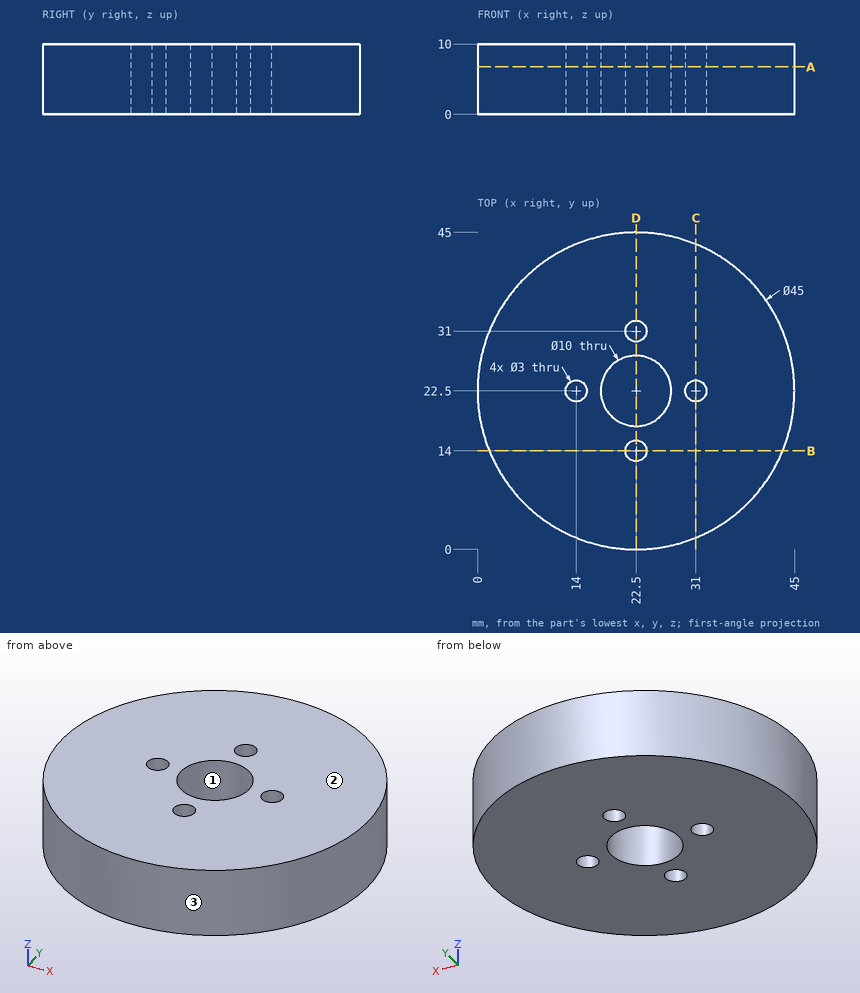
Geometry check sheet. Reference: drawing and pictorial views, mm from the part's lowest x, y, z. Give positions to 0.01 mm unless a question says otherwise; leave off trailing zeros. Order: outer loops, then holes, each group sorted by start corner. A loop starts at its lowest first (then second) coordinate and runs counter-clockwise, first axis right, second up. Notation, with made-up numbers: M 76,45 L 88,45 A21 cw 88,58 Z; hole C 17.25,39 d5. An arc over 180 degrees is marked long. Answer in a Markdown table with one row per item. Add a question column.
Item 1: Mould release check, pull along Y, two halves, no side actions. Record for the marked faces 1, 2 and 3: released by +Y, released by -Y, zero draft, split by the parting line, or undercut.
Item 2: Section check A-A, the plane z = 6.75. Enter the section's corners in (x, y), and give its area (3 significant figures).
Item 3: Gauge pin test, flat ends, axial feed: pin 1 (3.5 mm diameter, centred on x = 14, y = 22.5, fed in from +Z); pin 2 (3 mm diameter, centred on x = 17, z = 3.5, fed in from -Y); pin 3 (1.5 mm diameter, centred on y = 33, z = 7, fed in from -X); pin 4 (5 mm diameter, centred on y = 27, z = 5.5, fed in from -X). Record the tip position at first contact, or that the pin passes through.
Item 4: Section check B-B, the plane y = 14. Enter the section's corners in (x, z), and give its area (3 significant figures).
Item 5: Scan lines: probe 1 along Y at (x, z) = (22.5, 3.75); probe 2 along Y at (x, z) = (30.5, 0.5); probe 3 along Y at (x, z) = (14, 3.5). Record each from-to range of solid material in increasing order. Write a range as from..to.
Item 6: Section check D-D, the plane x = 22.5. Enter the section's corners in (y, z).
Filled sheet:
| question | item | result |
|---|---|---|
| 1 | face 1 | undercut |
| 1 | face 2 | zero draft |
| 1 | face 3 | split by the parting line |
| 2 | outline | C 22.5,22.5 d45; hole C 14,22.5 d3; hole C 22.5,22.5 d10; hole C 22.5,14 d3; hole C 22.5,31 d3; hole C 31,22.5 d3 |
| 2 | area | 1,480 mm^2 |
| 3 | pin 1 | stops at z = 10 |
| 3 | pin 2 | stops at y = 0.36 |
| 3 | pin 3 | stops at x = 2.22 |
| 3 | pin 4 | stops at x = 0.09 |
| 4 | outline | M 1.67,0 L 21,0 L 21,10 L 1.67,10 Z; M 24,0 L 43.33,0 L 43.33,10 L 24,10 Z |
| 4 | area | 387 mm^2 |
| 5 | probe 1 | y = 0..12.5, 15.5..17.5, 27.5..29.5, 32.5..45 |
| 5 | probe 2 | y = 1.47..21.09, 23.91..43.53 |
| 5 | probe 3 | y = 1.67..21, 24..43.33 |
| 6 | outline | M 0,0 L 12.5,0 L 12.5,10 L 0,10 Z; M 15.5,0 L 17.5,0 L 17.5,10 L 15.5,10 Z; M 27.5,0 L 29.5,0 L 29.5,10 L 27.5,10 Z; M 32.5,0 L 45,0 L 45,10 L 32.5,10 Z |
